```python
from build123d import *

# Parameters (mm, degrees)
BASE_EXTRUDE_DEPTH       = 14.2494
SKETCH2_R                = 3.175
SKETCH2_R_2              = 0.635
CUT_EXTRUDE1_DEPTH       = 11.7094
FILLET1_R                = 0.635
CUT_EXTRUDE2_DEPTH       = 10.8966
SKETCH4_W                = 0.508
SKETCH4_H                = 2.4892
SKETCH4_W_2              = 2.9972
SKETCH4_H_2              = 0.508
SKETCH4_W_3              = 2.4892
SKETCH4_H_3              = 0.254
BOSS_EXTRUDE1_DEPTH      = 3.683
BOSS_EXTRUDE1_DEPTH_BACK = 3.556
FILLET2_R                = 0.4572
CUT_EXTRUDE3_DEPTH       = 0.508
CUT_EXTRUDE4_DEPTH       = 0.508
CUT_EXTRUDE5_DEPTH       = 0.508


with BuildPart() as part:
    # Sketch1 → Base-Extrude (new body)
    with BuildSketch(Plane.XY):
        with BuildLine():
            Line((0.381, 0), (8.6106, 0))
            ThreePointArc((8.6106, 0), (8.880007684, 0.111592316), (8.9916, 0.381))
            Line((8.9916, 0.381), (8.9916, 10.5918))
            ThreePointArc((8.9916, 10.5918), (8.880007684, 10.861207684), (8.6106, 10.9728))
            Line((8.6106, 10.9728), (0.381, 10.9728))
            ThreePointArc((0.381, 10.9728), (0.111592316, 10.861207684), (0, 10.5918))
            Line((0, 10.5918), (0, 0.381))
            ThreePointArc((0, 0.381), (0.111592316, 0.111592316), (0.381, 0))
        make_face()
    extrude(amount=BASE_EXTRUDE_DEPTH)

    # Sketch2 → Cut-Extrude1 (cut)
    with BuildSketch(Plane.XY.offset(14.2494)):
        with Locations((4.4958, 6.477)):
            Circle(SKETCH2_R)
        with Locations((4.4958, 6.477)):
            Circle(SKETCH2_R_2, mode=Mode.SUBTRACT)
    extrude(amount=-CUT_EXTRUDE1_DEPTH, mode=Mode.SUBTRACT)

    # Fillet1
    fillet1_edges = [part.edges().sort_by_distance(p)[0] for p in [
        (3.8608, 6.477, 14.2494),
    ]]
    fillet(fillet1_edges, radius=FILLET1_R)

    # Sketch3 → Cut-Extrude2 (cut)
    with BuildSketch(Plane(origin=(0, 0, 0), x_dir=(-1, 0, 0), z_dir=(0, 0, -1))):
        with BuildLine():
            Line((-0.381, 10.9728), (-8.6106, 10.9728))
            ThreePointArc((-8.6106, 10.9728), (-8.880007684, 10.861207684), (-8.9916, 10.5918))
            Line((-8.9916, 10.5918), (-8.9916, 6.4516))
            ThreePointArc((-8.9916, 6.4516), (-4.4958, 10.9474), (0, 6.4516))
            Line((0, 6.4516), (0, 10.5918))
            ThreePointArc((0, 10.5918), (-0.111592316, 10.861207684), (-0.381, 10.9728))
        make_face()
    extrude(amount=-CUT_EXTRUDE2_DEPTH, mode=Mode.SUBTRACT)

    # Sketch4 → Boss-Extrude1 (add, two sides)
    with BuildSketch(Plane.XZ) as boss_extrude1_sk:
        with Locations((9.2202, 3.6322)):
            Rectangle(SKETCH4_W, SKETCH4_H)
        with Locations((4.4958, 0.635)):
            Rectangle(SKETCH4_W_2, SKETCH4_H_2)
        with Locations((4.4958, 6.8834)):
            Rectangle(SKETCH4_W_3, SKETCH4_H_3)
    extrude(amount=BOSS_EXTRUDE1_DEPTH)
    extrude(boss_extrude1_sk.sketch, amount=-BOSS_EXTRUDE1_DEPTH_BACK)

    # Fillet2
    fillet2_edges = [part.edges().sort_by_distance(p)[0] for p in [
        (9.4742, 3.556, 3.6322),
    ]]
    fillet(fillet2_edges, radius=FILLET2_R)

    # Sketch5 → Cut-Extrude3 (cut)
    with BuildSketch(Plane(origin=(0, 0, 0.381), x_dir=(-1, 0, 0), z_dir=(0, 0, -1))):
        with BuildLine():
            Line((-2.9972, -3.683), (-5.9944, -3.683))
            Line((-5.9944, -3.683), (-5.9944, -1.9304))
            ThreePointArc((-5.9944, -1.9304), (-4.4958, -3.429), (-2.9972, -1.9304))
            Line((-2.9972, -1.9304), (-2.9972, -3.683))
        make_face()
    extrude(amount=-CUT_EXTRUDE3_DEPTH, mode=Mode.SUBTRACT)

    # Sketch6 → Cut-Extrude4 (cut)
    with BuildSketch(Plane(origin=(0.312334932, -0.354120005, 6.7564), x_dir=(-1, 0, 0), z_dir=(0, 0, -1))):
        with BuildLine():
            Line((-2.938865068, -3.328879995), (-5.428065068, -3.328879995))
            Line((-5.428065068, -3.328879995), (-5.428065068, -1.830279995))
            ThreePointArc((-5.428065068, -1.830279995), (-4.183465068, -3.074879995), (-2.938865068, -1.830279995))
            Line((-2.938865068, -1.830279995), (-2.938865068, -3.328879995))
        make_face()
    extrude(amount=-CUT_EXTRUDE4_DEPTH, mode=Mode.SUBTRACT)

    # Sketch7 → Cut-Extrude5 (cut)
    with BuildSketch(Plane(origin=(9.4742, 0, 0), x_dir=(0, 0, -1), z_dir=(1, 0, 0))):
        with BuildLine():
            Line((-2.3876, -3.683), (-2.3876, -2.1844))
            ThreePointArc((-2.3876, -2.1844), (-3.6322, -3.429), (-4.8768, -2.1844))
            Line((-4.8768, -2.1844), (-4.8768, -3.683))
            Line((-4.8768, -3.683), (-2.3876, -3.683))
        make_face()
    extrude(amount=-CUT_EXTRUDE5_DEPTH, mode=Mode.SUBTRACT)


solid = part.part
```
Geometry check sheet. Reference: the model listing, model coordinates, mm. A direction names the side the tool comes from. Coordinates: 2 decimals unless noted, no trailing zeros. Order: outer loops, then holes, each group sorted by start corner. A loop starts at its lowest first (then second) coordinate and runs counter-clockwise, first axis right, second up.
Q1. Sectioned sample at D-D on z = 10.5. Record the cut outline in (x, y) (3 decimals).
Reply:
outline: (0, 0.381) arc R0.381 ccw to (0.381, 0) - (8.611, 0) arc R0.381 ccw to (8.992, 0.381) - (8.992, 6.452) arc R4.496 ccw to (0, 6.452) - close; circle Ø1.27 at (4.496, 6.477); hole circle Ø6.35 at (4.496, 6.477)
Q2. Sectioned sample at B-B on y = 1.5. Record the cut outline in (x, z), and give its area (3 significant figures).
Reply:
outline: (0, 0) - (8.99, 0) - (8.99, 2.39) - (9.47, 2.39) - (9.47, 4.88) - (8.99, 4.88) - (8.99, 14.25) - (0, 14.25) - close
area: 129 mm2
Q3. Depth check by flat-ended pin: pin 1 Ø1.5 at (x, z) = (1.5, 7.5) entering from +Y; pin 2 Ø5 at (x, z) = (5.5, 7) entering from +Y; pin 3 Ø2.5 at (x, y) = (5, -1.5) entering from +Z. Enter the tip coordinate at first touch or a pass-through.
Reply:
pin 1: stops at y = 10.35
pin 2: stops at y = 10.95
pin 3: stops at z = 7.01
Q4. Sectioned sample at C-C on x = 6.75. Record the cut outline in (y, z).
Reply:
outline: (0, 0) - (10.34, 0) - (10.34, 10.9) - (10.97, 10.9) - (10.97, 14.25) - (8.71, 14.25) - (8.71, 2.54) - (4.24, 2.54) - (4.24, 14.25) - (0, 14.25) - close
Q5. Draft check along X on faces 5 (the face through (4.358, 5.857, 8.155)), 6 (the face through (4, -2, 6.756)), 7 (the face through (4.595, 10.946, 5.372)), 8 (the face through (3.7, 6.5, 2.54)). Enter one of: released by +X, released by -X, zero draft, split by the parting line, or undercut.
Reply:
face 5: undercut
face 6: zero draft
face 7: split by the parting line
face 8: undercut
Q6. Thickness scan on probe 1 along Y at (x, z) = (4.5, 3.25); probe 2 along X at (y, z) = (6.25, 2.75); probe 3 along Z at (x, y) = (4.25, -1.5). Record the ranges inside material, lowest first.
Reply:
probe 1: y = 0 to 3.3, 5.84 to 7.11, 9.65 to 10.95
probe 2: x = 0 to 1.33, 3.9 to 5.09, 7.66 to 8.99
probe 3: z = 0.38 to 0.89, 6.76 to 7.01
Q7. Tool access check on faces 1 (the face through (4, -2, 0.889)), 2 (the face through (4, -2, 7.01)), 3 (the face through (6.5, 10.7, 10.897)), 4 (the face through (4, -2, 0.381)). Record the directions out of +Z, -Z, +X, -X, +Y, -Y that give a thin tool (end or side, any length) a straight path to the whole face; none if there is none.
Reply:
face 1: +X, -X, -Y
face 2: +Z, +X, -X, -Y
face 3: -Z, +Y
face 4: -Z, +X, -X, -Y
Q8. Sectioned sample at A-A on z = 4. Record the cut outline in (x, y) (3 decimals), and give its area (3 significant figures).
Reply:
outline: (0, 0.381) arc R0.381 ccw to (0.381, 0) - (8.611, 0) arc R0.381 ccw to (8.966, 0.244) - (8.966, -3.373) - (9.474, -3.373) - (9.474, 3.099) arc R0.457 ccw to (9.017, 3.556) - (8.992, 3.556) - (8.992, 6.452) arc R4.496 ccw to (0, 6.452) - close; circle Ø1.27 at (4.496, 6.477); hole circle Ø6.35 at (4.496, 6.477)
area: 62.7 mm2
